Verification items for the finished model (mm, model axes). Face numbers are marked on the shaded views. Coordinates: 2 decimals unless noted, no trailing zeros. Write each loop counter-clockwise with the first axis right and the second up, starting at its lowest first coordinate (ties: lowest second). Pieces come first, ordered by that corner, then holes. Notation, with made-up numbers: M 13.25,-12.5 L 69.25,-12.5 A23 cw 69.25,8.5 Z; hole C 26,41.5 d6. An arc over 180 degrees is marked long. Answer in a Markdown table with one row per item.
from build123d import *

# Parameters (mm, degrees)
BOSS_EXTRUDE1_DEPTH = 30
SKETCH1_3_W         = 100
SKETCH1_3_H         = 100
BOSS_EXTRUDE2_DEPTH = 1000


with BuildPart() as part:
    # Sketch1 → Boss-Extrude1 (new body)
    with BuildSketch(Plane(origin=(0, 0, 0), x_dir=(1, 0, 0), z_dir=(0, 1, 0))):
        Polygon((-400, -500), (400, -500), (400, -400), (500, -400), (500, 400), (400, 400), (400, 500), (-400, 500), (-400, 400), (-500, 400), (-500, -400), (-400, -400), align=None)
    extrude(amount=BOSS_EXTRUDE1_DEPTH)

    # Sketch1<3> → Boss-Extrude2 (add)
    with BuildSketch(Plane(origin=(0, 0, 0), x_dir=(1, 0, 0), z_dir=(0, 1, 0))):
        with Locations((-450, -450)):
            Rectangle(SKETCH1_3_W, SKETCH1_3_H)
        with Locations((-450, 450)):
            Rectangle(SKETCH1_3_W, SKETCH1_3_H)
        with Locations((450, 450)):
            Rectangle(SKETCH1_3_W, SKETCH1_3_H)
        with Locations((450, -450)):
            Rectangle(SKETCH1_3_W, SKETCH1_3_H)
    extrude(amount=BOSS_EXTRUDE2_DEPTH)


solid = part.part
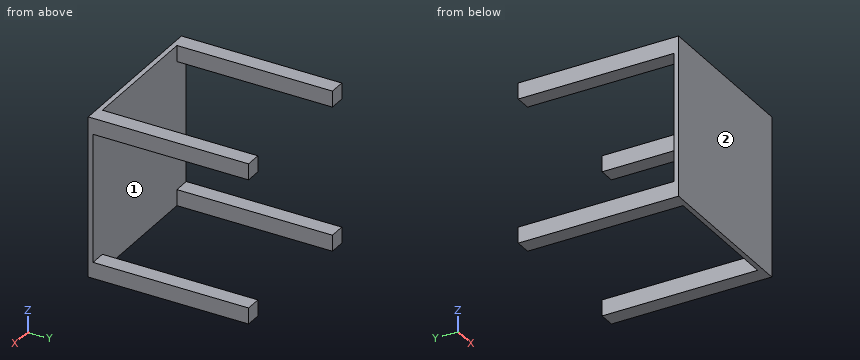
1) Thickness scan on L1, parallel to X at y = 793, z = 405; L2, parallel to Y at x = 182, z = 452.5. Record the ranges inside material, lowest first. Write a range as [from, to].
Response values:
| item | result |
|---|---|
| L1 | x = [-500, -400], [400, 500] |
| L2 | y = [0, 30] |
2) Sectioned sample at B-B (x = -326.5). Record the cut outline in (y, z).
Response values:
| item | result |
|---|---|
| outline | M 0,-500 L 30,-500 L 30,500 L 0,500 Z |
3) Sectioned sample at A-A (y = 534). Record the cut outline in (x, z).
Response values:
| item | result |
|---|---|
| outline | M -500,-500 L -400,-500 L -400,-400 L -500,-400 Z; M -500,400 L -400,400 L -400,500 L -500,500 Z; M 400,-500 L 500,-500 L 500,-400 L 400,-400 Z; M 400,400 L 500,400 L 500,500 L 400,500 Z |
4) Release check for a two-part mould opening along Z. For the marked faces 1 and 2 record: +Z half, -Z half, draft (parallel to the pull), parting line (faces both ways), or undercut.
Response values:
| item | result |
|---|---|
| face 1 | undercut |
| face 2 | draft |
5) Sectioned sample at C-C (z = 310.5). Record the cut outline in (x, y).
Response values:
| item | result |
|---|---|
| outline | M -500,0 L 500,0 L 500,30 L -500,30 Z |
6) Depth check by flat-ended pin: pin 1 (2 mm diameter, centred on x = -110, z = -114.5, fed in from +Y). Enter the tip coordinate at first touch or a pass-through.
Response values:
| item | result |
|---|---|
| pin 1 | stops at y = 30 |
